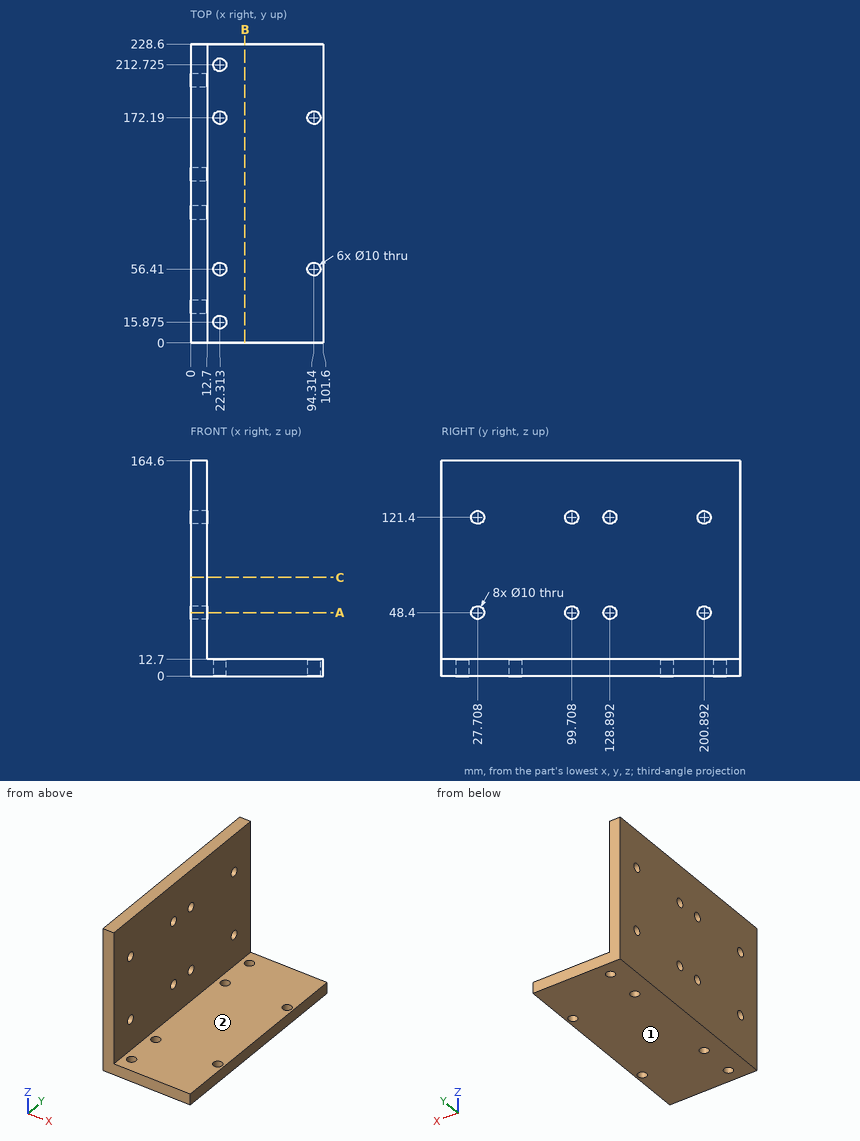
Could you check a few things on this drawing? It's one solid part, dimensions in mm from its lowest x, y, z. A direction names the side the tool comes from. Give positions to 0.01 mm unless a question says otherwise; leave off trailing zeros. Write each loop counter-clockwise with the first axis right and the second up, starting at its lowest first coordinate (ties: lowest second). Pieces come first, ordered by that corner, then holes. Notation, with made-up numbers: (-39, 9.5) - (-24, 9.5) arc R17 ccw to (-24, 36.5) - close; hole circle Ø8 at (-32, 64.5). An arc over 180 degrees is marked (long way). Use CSV: the item, a comma, the result in double quotes. Start each with the question number.
Item 1: If I drill on line 1 along Y through (x, z) = (9, 48); line 2 along Z through (x, y) = (16, 36), over which ranges is the centre line in solid material (lowest first)?
Item 2: I want a section at A-A, the plane z = 48.4. Please give me the cut outline in (x, y).
Item 3: I'm going to push flat-ended pins straight in: pin 1 (10 mm diameter, centred on y = 77, z = 74.5, fed in from +X); pin 2 (13 mm diameter, centred on x = 22.31, y = 172.19, fed in from +Z); pin 3 (8 mm diameter, centred on y = 99.708, z = 48.4, fed in from -X). Where does each tip first touch, or does it pass through?
Item 4: I want a section at B-B, the plane x = 41.5. Please give me the cut outline in (y, z), then the cut area to 3 significant figures.
Item 5: I want a section at C-C, the plane z = 75.5. Please give me the cut outline in (x, y), then the cut area to 3 significant figures.
Item 6: For the marked faces 1 and 2, which set-ups out of +Z, -Z, +X, -X, +Y, -Y let a thin tool reach every point of the face, with its end or its side?
Findings:
1,line 1,"y = 0 to 22.72, 32.69 to 94.72, 104.69 to 123.91, 133.88 to 195.91, 205.88 to 228.6"
1,line 2,"z = 0 to 12.7"
2,outline,"(0, 0) - (12.7, 0) - (12.7, 22.71) - (0, 22.71) - close; (0, 32.71) - (12.7, 32.71) - (12.7, 94.71) - (0, 94.71) - close; (0, 104.71) - (12.7, 104.71) - (12.7, 123.89) - (0, 123.89) - close; (0, 133.89) - (12.7, 133.89) - (12.7, 195.89) - (0, 195.89) - close; (0, 205.89) - (12.7, 205.89) - (12.7, 228.6) - (0, 228.6) - close"
3,pin 1,"stops at x = 12.7"
3,pin 2,"stops at z = 12.7"
3,pin 3,"passes through"
4,outline,"(0, 0) - (228.6, 0) - (228.6, 12.7) - (0, 12.7) - close"
4,area,"2,900 mm2"
5,outline,"(0, 0) - (12.7, 0) - (12.7, 228.6) - (0, 228.6) - close"
5,area,"2,900 mm2"
6,face 1,"-Z, +X, -X, +Y, -Y"
6,face 2,"+Z, +X, +Y, -Y"
